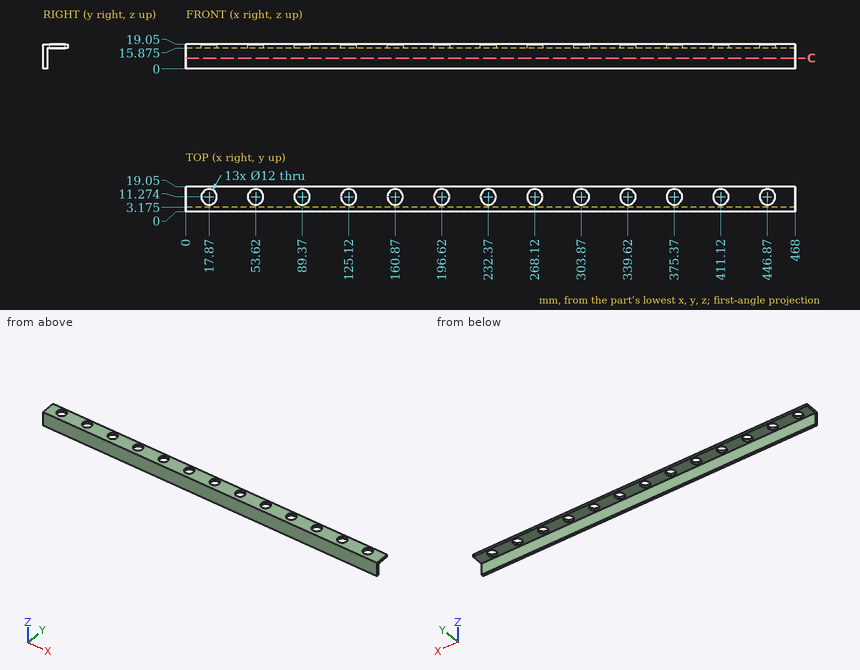
Input: dimensioned drawing with shaded views. Units: mm. Origin: part minimum x, y, z. Round coordinates to 2 decimals unless told otherwise and drop trailing zeros. Loops run counter-clockwise (first coordinate to the right, second up) from the corner with the lowest first, then second, coordinate; pieces in that order, holes last.
1) Pin query (flat end, axial travel): pin 1 (6 mm diameter, centred on x = 179, z = 2.5, fed in from +Y) (3 decimals). Return the tip coordinate at first contact, or that it passes through.
Ans:
pin 1: stops at y = 3.175
2) Material intervals for line 1 (Y direction, x = 160.87, z = 17.6); line 2 (Y direction, x = 85.5, z = 9.5) (1 decimal); line 3 (Y direction, x = 161.5, z = 16.75), sorted ascending.
Ans:
line 1: y = 0 to 5.27, 17.27 to 19.05
line 2: y = 0 to 3.2
line 3: y = 0 to 5.31, 17.24 to 19.05
3) Section query C-C on z = 8.25. Return the cut outline in (x, y) (1 decimal), plus the area to 3 significant figures.
Ans:
outline: (0, 0) - (468, 0) - (468, 3.2) - (0, 3.2) - close
area: 1,490 mm2
